Build history of the part. All positions in model axes, mm. Round coordinates to 2 decimals unless told otherwise and drop trailing zeros. Order: outer loops, then holes, each group sorted by start corner. A loop starts at its lowest first (then second) coordinate and runs counter-clockwise, first axis right, second up. Notation, with made-up numbers: M 77.5,-31 L 96.5,-31 A21 ccw 96.5,-10 Z; hole C -23.75,16.5 d6. An arc over 180 degrees is marked long. One line per item, written item: value. Start each with the question number.
Item 1: Band-saw the part on B-B, the plane x = 7.5. Write the cut outline in (y, z), then the cut area to 3 significant figures.
Item 2: Probe L1, parallel to Z at x = 37, y = -19; L2, parallel to Z at x = -1.5, y = -11; L3, parallel to X at y = -15.5, z = -9.5. List the from-to ranges inside material, lowest first.
Item 3: Band-saw the part on D-D, the plane y = -40. Write the cut outline in (x, z), then the cut area to 3 significant figures.
Item 4: Band-saw the part on A-A, the plane y = -69. Write the cut outline in (x, z), then the cut area to 3 significant figures.
Item 5: Pin check, flat tips, straight feed: pin 1 (5 mm diameter, centred on y = -63.5, z = -3.5, fed in from +X); pin 2 (12 mm diameter, centred on x = 37.5, z = -37.5, fed in from -Y); pin 3 (4 mm diameter, centred on x = -6.5, z = 30, fed in from +Y). Stop position of each tip, or through.
Item 6: Band-saw the part on C-C, the plane z = -7.5. Write the cut outline in (x, y), then the cut area to 3 significant figures.
```python
from build123d import *

# Parameters (mm, degrees)
F1_ANGLE = 180
F2_T     = -2.5
F4_W     = 39.3107756972
F4_H     = 39.0258319676


with BuildPart() as f1:
    # F0 (on Front) → F1 (revolve)
    with BuildSketch(Plane.XZ):
        with BuildLine():
            ThreePointArc((0, -53.6816862102), (37.9586843448, -37.9586843448), (53.6816862102, 0))
            ThreePointArc((53.6816862102, 0), (37.9586843448, 37.9586843448), (0, 53.6816862102))
            Line((0, 53.6816862102), (0, -53.6816862102))
        make_face()
    revolve(axis=Axis((0, 0, 0), (0, 0, -1)), revolution_arc=F1_ANGLE)

    # F2
    f2_openings = [f1.faces().sort_by_distance(p)[0] for p in [
        (0, 0, 0),
    ]]
    offset(amount=F2_T, openings=f2_openings)

    # F4 (on offset) → F5 (join, up to the next surface of F1)
    with BuildSketch(Plane.XZ.offset(80)):
        Rectangle(F4_W, F4_H)
    extrude(until=Until.NEXT, dir=(0, 1, 0))


solid = f1.part
```
Output:
1. outline: M -80,-19.51 L -49.44,-19.51 A53.16 ccw 0,-53.16 L 0,-50.63 A50.63 cw 0,50.63 L 0,53.16 A53.16 ccw -49.44,19.51 L -80,19.51 Z
1. area: 1,510 mm²
2. L1: z = -33.94 to -29.83, 29.83 to 33.94
2. L2: z = -52.52 to -49.96, 49.96 to 52.52
2. L3: x = -50.51 to -47.84, 47.84 to 50.51
3. outline: C 0,0 d71.6; hole C 0,0 d63.86
3. area: 824 mm²
4. outline: M -19.66,-19.51 L 19.66,-19.51 L 19.66,19.51 L -19.66,19.51 Z
4. area: 1,530 mm²
5. pin 1: stops at x = 19.66
5. pin 2: stops at y = -25.88
5. pin 3: stops at y = -39.38
6. outline: M -53.16,0 A53.16 ccw -19.66,-49.39 L -19.66,-80 L 19.66,-80 L 19.66,-49.39 A53.16 ccw 53.16,0 L 50.63,0 A50.63 cw -50.63,0 Z
6. area: 1,520 mm²
